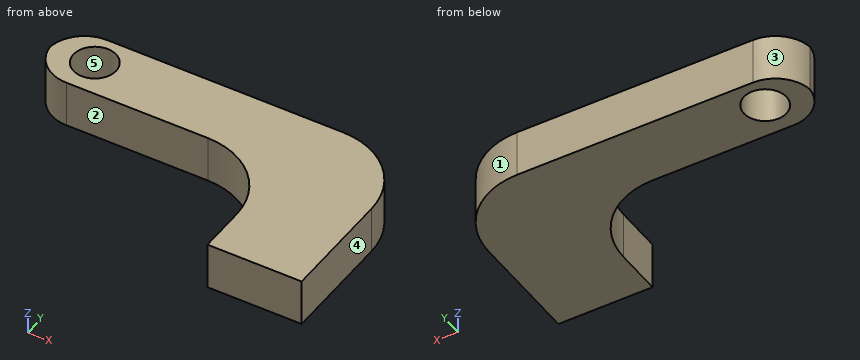
```python
from build123d import *

# Parameters (mm, degrees)
SKETCH1_R           = 2.8702
BOSS_EXTRUDE1_DEPTH = 6.35
FILLET1_R           = 10
FILLET2_R           = 5


with BuildPart() as part:
    # Sketch1 → Boss-Extrude1 (new body)
    with BuildSketch(Plane.XY):
        Polygon((-12.7, 38.1), (-25.4, 38.1), (-25.4, 44.45), (-25.4, 54.5), (-59.481100474, 54.5), (-59.481100474, 63.5), (-12.7, 63.5), (-12.7, 54.424612003), (-12.7, 44.45), align=None)
        with Locations((-53.575, 59.289941788)):
            Circle(SKETCH1_R, mode=Mode.SUBTRACT)
    extrude(amount=BOSS_EXTRUDE1_DEPTH)

    # Fillet1
    fillet1_edges = [part.edges().sort_by_distance(p)[0] for p in [
        (-25.4, 54.5, 3.175),
        (-12.7, 63.5, 3.175),
    ]]
    fillet(fillet1_edges, radius=FILLET1_R)

    # Fillet2
    # the kernel refuses this fillet: 5 mm, written as the material it takes off along each edge
    with BuildSketch(Plane(origin=(-59.481100474, 63.5, -12.5), x_dir=(0, -1, 0), z_dir=(0, 0, 1)), Plane(origin=(-59.481100474, 54.5, -12.5), x_dir=(1, 0, 0), z_dir=(0, 0, 1))) as fillet2_piece_1:
        with BuildLine():
            CenterArc((FILLET2_R, FILLET2_R), FILLET2_R, 180, 90)
            Line((0, FILLET2_R), (0, 0))
            Line((0, 0), (FILLET2_R, 0))
        make_face()
    extrude(amount=31.35, mode=Mode.SUBTRACT)


solid = part.part
```
Work out the finished part from the listing and answer in its coordinate system (mm). Face numbers are marked on the shaded views. A direction names the side the tool comes from. Coordinates: 2 decimals unless noted, no trailing zeros. Order: outer loops, then holes, each group sorted by start corner. A loop starts at its lowest first (then second) coordinate and runs counter-clockwise, first axis right, second up. Notation, with made-up numbers: (41.25, 50) - (94.25, 50) arc R28 cw to (94.25, 84) - close; hole circle Ø10 at (61, 36). An arc over 180 degrees is marked (long way). Answer as a JSON object with one key per item and string values.
1. A tool of negligible diameter and unlimited length cuts with its end or side. For the marked faces 1 and 2, from which of +Z, -Z, +X, -X, +Y, -Y can it reach the whole face along a straight path? Write none if from no direction.
Output values:
{"face 1": "+Z, -Z, +X, +Y", "face 2": "+Z, -Z, -X, -Y"}
2. Consider line 1 (Y direction, x = -47.5, z = 1); line 2 (X direction, y = 61.75, z = 6); line 3 (X direction, y = 57, z = 4.5). Determine where each line is inside the solid, lowest interval first.
Output values:
{"line 1": "y = 54.5 to 63.5", "line 2": "x = -58.28 to -55.05, -52.1 to -17.05", "line 3": "x = -58.81 to -55.31, -51.84 to -13.33"}
3. Find section A-A on y = 61. Determine the outline of the cut face in (x, z), plus the area to 3 significant figures.
Output values:
{"outline": "(-58.81, 0) - (-55.88, 0) - (-55.88, 6.35) - (-58.81, 6.35) - close; (-51.27, 0) - (-16.09, 0) - (-16.09, 6.35) - (-51.27, 6.35) - close", "area": "242 mm²"}
4. Find section C-C on x = -42. Determine the outline of the cut face in (y, z), plus the area to 4 significant figures.
Output values:
{"outline": "(54.5, 0) - (63.5, 0) - (63.5, 6.35) - (54.5, 6.35) - close", "area": "57.15 mm²"}
5. Each of these flat-tipped pins is pushed along its axis until it touches: P1, Ø1.5, axis at x = -29.5, z = 2.5, coming from the -Y side; P2, Ø3, axis at y = 40, z = 4.5, coming from the -X side; P3, Ø1.5, axis at y = 54.5, z = 5, coming from the -X side (3 decimals). Where does it stop, or does it pass through?
Output values:
{"P1": "stops at y = 51.97", "P2": "stops at x = -25.4", "P3": "stops at x = -57.115"}
6. Find section D-D on y = 46.25. Determine the outline of the cut face in (x, z), plus the area to 3 significant figures.
Output values:
{"outline": "(-25.55, 0) - (-12.7, 0) - (-12.7, 6.35) - (-25.55, 6.35) - close", "area": "81.6 mm²"}
7. Find section B-B on z = 5.75. Determine the outline of the cut face in (x, y) (3 decimals), plus the area to 3 significant figures.
Output values:
{"outline": "(-59.456, 59) arc R5 ccw to (-54.481, 54.5) - (-35.4, 54.5) arc R10 cw to (-25.4, 44.5) - (-25.4, 38.1) - (-12.7, 38.1) - (-12.7, 53.5) arc R10 ccw to (-22.7, 63.5) - (-54.481, 63.5) arc R5 ccw to start; hole circle Ø5.74 at (-53.575, 59.29)", "area": "593 mm²"}
8. The mould has two halves that part along X. Classify the marked faces 3, 4 and 5: +X half, -X half, draft (parallel to the pull), parting line (faces both ways), or undercut.
Output values:
{"face 3": "-X half", "face 4": "+X half", "face 5": "undercut"}
